Geometry check sheet. Reference: the model listing, model coordinates, mm. Face numbers are marked on the shaded views. A direction names the side the tool comes from. Round coordinates to 2 decimals unless told otherwise and drop trailing zeros. Write each loop counter-clockwise with the first axis right and the second up, starting at its lowest first coordinate (ties: lowest second). Pieces come first, ordered by that corner, then holes. Notation, with made-up numbers: (10, 82.25) -> (48, 82.25) arc R28 ccw to (48, 101.25) -> close; hole circle Ø10 at (-23, 57.25). An arc over 180 degrees is marked (long way). One line per question, with ' | ' between items.
Autodesk Inventor part; units mm, degrees
ref_plane "YZ Plane" through (0, 0, 0) normal (1, 0, 0) x (0, 1, 0)
ref_plane "XZ Plane" through (0, 0, 0) normal (0, 1, 0) x (-1, 0, 0)
ref_plane "XY Plane" through (0, 0, 0) normal (0, 0, 1) x (1, 0, 0)
sketch "Sketch2" plane through (0, 0, 0) normal (1, 0, 0) x (0, 1, 0)
  line L0 (0, 0) -> (0, -19.05)
  line L1 (0, -19.05) -> (44.45, -19.05)
  line L2 (44.45, -19.05) -> (44.45, -9.652)
  line L3 (44.45, -9.652) -> (9.525, -9.652)
  line L4 (9.525, -9.652) -> (9.525, 0)
  line L5 (9.525, 0) -> (0, 0) construction
  line L6 (0, 0) -> (0, 19.05)
  line L7 (0, 19.05) -> (44.45, 19.05)
  line L8 (44.45, 19.05) -> (44.45, 9.652)
  line L9 (44.45, 9.652) -> (9.525, 9.652)
  line L10 (9.525, 9.652) -> (9.525, 0)
  dimension "d5" = 44.45
  dimension "d7" = 9.398
  dimension "d8" = 9.525
  dimension "d42" = 9.652
extrude "Extrusion2" add sketch "Sketch2" along normal mid plane 44.45
sketch "Sketch3" plane through (-22.225, 0, 19.05) normal (0, 0, 1) x (1, 0, 0)
  line L0 (0, 44.45) -> (44.45, 44.45)
  line L1 (22.225, 44.45) -> (22.225, 0) construction
  point P0 (22.225, 34.925)
  dimension "d19" = 9.525
hole "Hole2" at (0, 34.925, 19.05) direction (0, 0, -1) diameter 6.7564 end through all
sketch "Sketch4" plane through (-22.225, 0, -19.05) normal (0, -1, 0) x (1, 0, 0)
  line L0 (44.45, 9.398) -> (44.45, 28.702) construction
  line L1 (44.45, 19.05) -> (0, 19.05) construction
  line L2 (0, 28.702) -> (0, 9.398) construction
  line L3 (44.45, 38.1) -> (44.45, 0) construction
  line L4 (19.05, 19.05) -> (-25.4, 19.05) construction
  point P0 (22.225, 19.05)
  point P1 (34.925, 19.05)
  point P2 (9.525, 19.05)
  dimension "d27" = 9.525
  dimension "d30" = 25.4
hole "Hole3" at (12.7, 0, 0) at (-12.7, 0, 0) direction (0, 1, 0) diameter 6.7564 end through all
properties part number "BracketForEndOfArm"
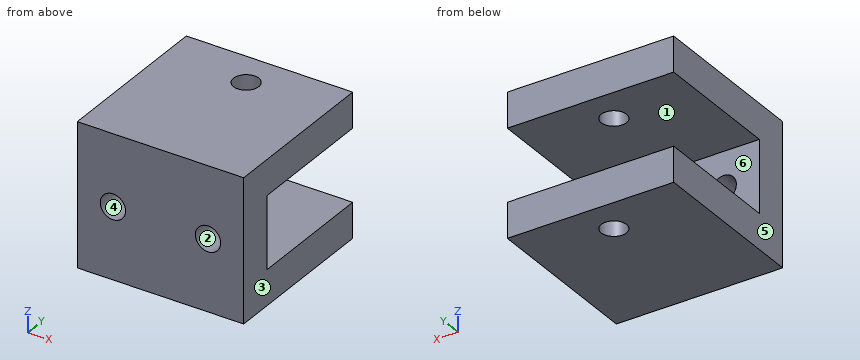
(1) Access from +Z, -Z, +X, -X, +Y, -Y to the whole of each face (thin tool, end or side, straight path). Record for the marked faces 1 and 2.
Resolved:
face 1: +X, -X, +Y | face 2: +Y, -Y
(2) Sectioned sample at B-B on y = 14. Record the cut outline in (x, z) (3 decimals).
Resolved:
outline: (-22.225, -19.05) -> (22.225, -19.05) -> (22.225, -9.652) -> (-22.225, -9.652) -> close; (-22.225, 9.652) -> (22.225, 9.652) -> (22.225, 19.05) -> (-22.225, 19.05) -> close
(3) Draft check along X on the marked faces 3, 4, 5 and 6. Enter one of: +X half, -X half, draft (parallel to the pull), parting line (faces both ways), or undercut.
Resolved:
face 3: +X half | face 4: undercut | face 5: -X half | face 6: draft
(4) Go/stop test with flat-tipped pins: pin 1 (9.5 mm diameter, centred on x = -8.5, z = 3, fed in from +Y) (3 decimals); pin 2 (4 mm diameter, centred on x = 12.7, z = 0, fed in from +Y). Record where each tip stops, or that it passes through.
Resolved:
pin 1: stops at y = 9.525 | pin 2: passes through
(5) Sectioned sample at C-C on z = 0. Record the cut outline in (x, y) (3 decimals).
Resolved:
outline: (-22.225, 0) -> (-16.078, 0) -> (-16.078, 9.525) -> (-22.225, 9.525) -> close; (-9.322, 0) -> (9.322, 0) -> (9.322, 9.525) -> (-9.322, 9.525) -> close; (16.078, 0) -> (22.225, 0) -> (22.225, 9.525) -> (16.078, 9.525) -> close
(6) Sectioned sample at A-A on x = 0. Record the cut outline in (y, z) (3 decimals), then the cut area to 3 significant figures.
Resolved:
outline: (0, -19.05) -> (31.547, -19.05) -> (31.547, -9.652) -> (9.525, -9.652) -> (9.525, 9.652) -> (31.547, 9.652) -> (31.547, 19.05) -> (0, 19.05) -> close; (38.303, -19.05) -> (44.45, -19.05) -> (44.45, -9.652) -> (38.303, -9.652) -> close; (38.303, 9.652) -> (44.45, 9.652) -> (44.45, 19.05) -> (38.303, 19.05) -> close | area: 892 mm2
(7) Material ranges on line 1 (X direction, y = 7.5, z = 0) (3 decimals); line 2 (Z direction, x = -2, y = 19); line 3 (Z direction, x = 12.7, y = 6.25), recorded low to high.
Resolved:
line 1: x = -22.225 to -16.078, -9.322 to 9.322, 16.078 to 22.225 | line 2: z = -19.05 to -9.65, 9.65 to 19.05 | line 3: z = -19.05 to -3.38, 3.38 to 19.05
(8) Sectioned sample at D-D on x = -12.7. Record the cut outline in (y, z) (3 decimals).
Resolved:
outline: (0, -19.05) -> (44.45, -19.05) -> (44.45, -9.652) -> (9.525, -9.652) -> (9.525, -3.378) -> (0, -3.378) -> close; (0, 3.378) -> (9.525, 3.378) -> (9.525, 9.652) -> (44.45, 9.652) -> (44.45, 19.05) -> (0, 19.05) -> close
